Design review of the part built by this model. Coordinates are the model's own, in mm. A direction names the side the tool comes from. Coordinates: 2 decimals unless noted, no trailing zeros. Write each loop counter-clockwise with the first axis right and the second up, starting at its lowest first coordinate (ties: lowest second). Pieces come first, ordered by that corner, then holes. Notation, with made-up numbers: M -39,22 L -7,22 A24 ccw -7,45 Z; hole C 42.5,9 d6. An arc over 180 degrees is marked long. Return JSON: item names as keys, results as strings. Group by question number.
```python
from build123d import *

# Parameters (mm, degrees)
SKETCH1_R       = 5.6896
EXTRUDE3_DEPTH  = 3.2512
SKETCH4_W       = 19.05
SKETCH4_H       = 2.413
CHAMFER2_SIZE   = 0.5953125
SKETCH26_R      = 0.5461
EXTRUDE13_DEPTH = 3.229849154


with BuildPart() as part:
    # Sketch1 → Extrude3 (new body)
    with BuildSketch(Plane.XY):
        Circle(SKETCH1_R)
    extrude(amount=EXTRUDE3_DEPTH)

    # Sketch11 → Cut-Revolve3 (revolve, cut)
    with BuildSketch(Plane(origin=(0, 0, 0), x_dir=(0, 0, -1), z_dir=(1, 0, 0))):
        with BuildLine():
            Line((-3.5052, 6.82752), (0, 6.82752))
            Line((0, 6.82752), (0, 5.6896))
            Line((0, 5.6896), (-0.32512, 5.6896))
            ThreePointArc((-0.32512, 5.6896), (-2.476812954, 3.198964376), (-3.2512, 0))
            Line((-3.2512, 0), (-3.5052, 0))
            Line((-3.5052, 0), (-3.5052, 6.82752))
        make_face()
    revolve(axis=Axis((0, 0, 0), (0, 0, 1)), mode=Mode.SUBTRACT)



with BuildPart() as body_2:
    # Sketch4 → Revolve1 (revolve)
    with BuildSketch(Plane(origin=(0, 0, 0), x_dir=(0, 0, -1), z_dir=(1, 0, 0))):
        with Locations((9.525, 1.2065)):
            Rectangle(SKETCH4_W, SKETCH4_H)
    revolve(axis=Axis((0, 0, 0), (0, 0, -1)))

    # Chamfer2
    chamfer2_edges = [body_2.edges().sort_by_distance(p)[0] for p in [
        (0, -2.413, -19.05),
    ]]
    chamfer(chamfer2_edges, length=CHAMFER2_SIZE)


with BuildPart() as part_1:
    add(part.part)

    add(body_2.part)  # Extrude13 merges body 2
    # Sketch26 → Extrude13 (add)
    with BuildSketch(Plane.XY):
        Circle(SKETCH26_R)
    extrude(amount=EXTRUDE13_DEPTH)


solid = part_1.part
```
Item 1: For pin 1 (3 mm diameter, centred on x = -4, y = 1, fed in from +Z); pin 2 (4 mm diameter, centred on y = -3.5, z = -4.5, fed in from +X); pin 3 (1.5 mm diameter, centred on x = -4.5, y = 0, fed in from +Z), all flat-tipped, find the tip position at first contact; note any pin that passes through.
Item 2: Add section D-D (y = 3.5). Write out the cut boundary in (x, z).
Item 3: Add section A-A (y = 0). Write out the cut boundary in (x, z), plus the area to 3 significant figures.
Item 4: Add section C-C (z = -2.25). Write out the cut boundary in (x, y).
Item 5: Machinability: for faces 1 (the cylindrical face through (-1.468, -1.915, -9.357)), 2 (the flat face through (0, 0, -19.05)), which of the approach directions +Z, -Z, +X, -X, +Y, -Y give a long, thin tool a straight path to every point of the face, cutting with its end or side? Answer none if there is none.
Item 6: For line 1 (Z direction, x = 1, y = 4.5); line 2 (Y direction, x = 1.5, z = -5.75); line 3 (Z direction, x = 1.75, y = 3), list the stretches that pass through material, from the lowest coordinate up.
Geometry check:
{
 "1": {"pin 1": "z = 2.74", "pin 2": "x = 1.89", "pin 3": "z = 2.16"},
 "2": {"outline": "M -4.49,0 L 4.49,0 L 4.49,0.33 A6.06 ccw -4.49,0.33 Z"},
 "3": {"outline": "M -5.69,0 L -2.41,0 L -2.41,-18.45 L -1.82,-19.05 L 1.82,-19.05 L 2.41,-18.45 L 2.41,0 L 5.69,0 L 5.69,0.33 A6.99 ccw -5.69,0.33 Z", "area": "119 mm^2"},
 "4": {"outline": "C 0,0 d4.83"},
 "5": {"face 1": "-Z", "face 2": "-Z, +X, -X, +Y, -Y"},
 "6": {"line 1": "0 to 1.52", "line 2": "-1.89 to 1.89", "line 3": "0 to 2.33"}
}
